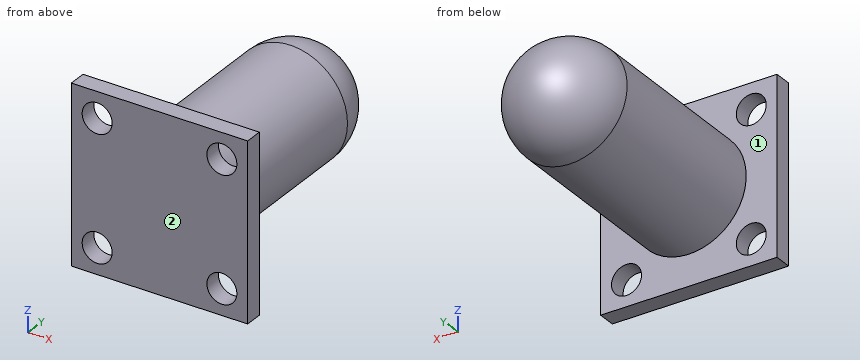
```python
from build123d import *

# Parameters (mm, degrees)
ESQUISSE3_W          = 20
ESQUISSE3_H          = 20
BOSS_EXTRU_1_DEPTH   = 2
D_GAGEMENT_M31_D     = 3.4
D_GAGEMENT_M31_DEPTH = 3
D_GAGEMENT_M31_TIP   = 1.021463052


with BuildPart() as part:
    # Esquisse2 → Révolution3 (revolve)
    with BuildSketch(Plane.XY):
        with BuildLine():
            Line((4, 0), (6.5, 0))
            Line((6.5, 0), (6.5, 20.5))
            ThreePointArc((6.5, 20.5), (4.596194078, 25.096194078), (0, 27))
            Line((0, 27), (0, 25.944271904))
            Line((0, 25.944271904), (0, 24.5))
            ThreePointArc((0, 24.5), (2.828427125, 23.328427125), (4, 20.5))
            Line((4, 20.5), (4, 0))
        make_face()
    revolve(axis=Axis((0, 0, 0), (0, 1, 0)))

    # Esquisse3 → Boss.-Extru.1 (add)
    with BuildSketch(Plane.XZ):
        Rectangle(ESQUISSE3_W, ESQUISSE3_H)
    extrude(amount=BOSS_EXTRU_1_DEPTH)

    # Dégagement M31
    with Locations(Plane(origin=(0, 0, 0), x_dir=(1, 0, 0), z_dir=(0, 1, 0))):
        with Locations((-7.071067812, 7.071067812), (7.071067812, 7.071067812), (7.071067812, -7.071067812), (-7.071067812, -7.071067812)):
            Hole(D_GAGEMENT_M31_D / 2, depth=D_GAGEMENT_M31_DEPTH)
            with Locations((0, 0, -(D_GAGEMENT_M31_DEPTH + D_GAGEMENT_M31_TIP / 2))):  # 118° drill point
                Cone(0, D_GAGEMENT_M31_D / 2, D_GAGEMENT_M31_TIP, mode=Mode.SUBTRACT)


solid = part.part
```
Could you check a few things on this model? Use its own coordinates, in mm. Face numbers are marked on the shaded views. A direction names the side the tool comes from. Give positions to 0.01 mm unless a question says otherwise; leave off trailing zeros. Loops run counter-clockwise (first coordinate to the right, second up) from the corner with the lowest first, then second, coordinate; pieces in that order, holes last. Notation, with made-up numbers: (67, 9) - (120, 9) arc R19 ccw to (120, 27) - close; hole circle Ø2 at (-19.5, 10.5). An arc over 180 degrees is marked (long way). Use one line per item in the form item = value.
1. I need wall thicknesses on probe 1 along Z at (x, y) = (0, 17.5); probe 2 along X at (y, z) = (14, 1); probe 3 along Y at (x, z) = (-0.25, 7.5). Which ranges of each line are inside material? Lowest first, please.
Response values:
probe_1 = -6.5 to -4, 4 to 6.5
probe_2 = -6.42 to -3.87, 3.87 to 6.42
probe_3 = -2 to 0
2. I want a section at C-C (x = 8). Please give me the cut outline in (y, z).
Response values:
outline = (-2, -10) - (0, -10) - (0, -8.49) - (-2, -8.49) - close; (-2, -5.65) - (0, -5.65) - (0, 5.65) - (-2, 5.65) - close; (-2, 8.49) - (0, 8.49) - (0, 10) - (-2, 10) - close
3. I want a section at D-D (y = 12). Please give me the cut outline in (x, z).
Response values:
outline = circle Ø13 at (0, 0); hole circle Ø8 at (0, 0)
4. On a 3-axis mill with a long thin cutter (end or side, diameter ignored), from which of +Z, -Z, +X, -X, +Y, -Y can I reach the whole of each face in a straight line? I mean the marked faces 1 and 2. Say none if no direction works.
Response values:
face_1 = +Y
face_2 = +Z, -Z, +X, -X, -Y
5. I want a section at B-B (x = 0). Please give me the cut outline in (y, z).
Response values:
outline = (-2, -10) - (0, -10) - (0, -6.5) - (20.5, -6.5) arc R6.5 ccw to (20.5, 6.5) - (0, 6.5) - (0, 10) - (-2, 10) - close; hole (0, -4) - (20.5, -4) arc R4 ccw to (20.5, 4) - (0, 4) - close
6. I'm going to push flat-ended pins straight in: pin 1 Ø2 at (y, z) = (6, -3.5) entering from -X; pin 2 Ø4 at (x, z) = (-7.5, 5) entering from +Y; pin 3 Ø2 at (x, z) = (-3.5, -6) entering from +Y. Where does each tip first touch, or does it pass through?
Response values:
pin_1 = -6
pin_2 = 0
pin_3 = 23.13
7. I want a section at A-A (z = 0). Please give me the cut outline in (x, y).
Response values:
outline = (-10, -2) - (10, -2) - (10, 0) - (6.5, 0) - (6.5, 20.5) arc R6.5 ccw to (-6.5, 20.5) - (-6.5, 0) - (-10, 0) - close; hole (-4, 0) - (4, 0) - (4, 20.5) arc R4 ccw to (-4, 20.5) - close
